Here's how the part is built. I have some questions about the finished solid (model axes, mm). Face numbers are marked on the shaded views. A direction names the side the tool comes from. Round coordinates to 2 decimals unless told otherwise and drop trailing zeros. Loops run counter-clockwise (first coordinate to the right, second up) from the corner with the lowest first, then second, coordinate; pieces in that order, holes last. Notation, with made-up numbers: M -16.75,5.5 L 11.25,5.5 A6 cw 11.25,13.5 Z; hole C 62.25,4 d10. An arc over 180 degrees is marked long. Answer as CSV lines item,"result".
```python
from build123d import *

# Parameters (mm, degrees)
F2_DEPTH = 12.7
F1_R     = 4.7625
F1_R_2   = 1.5875
F3_DEPTH = 9.525
F4_R     = 1.5875
F5_DEPTH = 15.859309


with BuildPart() as f2:
    # F0 (on Top) → F2 (new body)
    with BuildSketch(Plane.XY):
        with BuildLine():
            Line((-5.552635, 5.67205), (-5.552635, 8.681886))
            ThreePointArc((-5.552635, 8.681886), (0, -10.305673), (5.552635, 8.681886))
            Line((5.552635, 8.681886), (5.552635, 5.67205))
            ThreePointArc((5.552635, 5.67205), (7.317033, 3.076513), (7.9375, 0))
            ThreePointArc((7.9375, 0), (-3.076513, -7.317033), (-5.552635, 5.67205))
        make_face()
        with BuildLine():
            Line((-5.552635, 23.249359), (-5.552635, 8.681886))
            Line((-5.552635, 8.681886), (-5.552635, 5.67205))
            ThreePointArc((-5.552635, 5.67205), (-4.520661, 6.52438), (-3.360147, 7.191197))
            Line((-3.360147, 7.191197), (-3.360147, 23.249359))
            Line((-3.360147, 23.249359), (-5.552635, 23.249359))
        make_face()
        with BuildLine():
            Line((5.552635, 5.67205), (5.552635, 8.681886))
            Line((5.552635, 8.681886), (5.552635, 23.249359))
            Line((5.552635, 23.249359), (3.360147, 23.249359))
            Line((3.360147, 23.249359), (3.360147, 7.191197))
            ThreePointArc((3.360147, 7.191197), (4.520661, 6.52438), (5.552635, 5.67205))
        make_face()
    extrude(amount=F2_DEPTH)

    # F1 (on Right) → F3 (join, symmetric)
    with BuildSketch(Plane.YZ):
        with Locations((-12.700004, 4.7625)):
            Circle(F1_R)
        with Locations((-12.700004, 4.7625)):
            Circle(F1_R_2, mode=Mode.SUBTRACT)
    extrude(amount=F3_DEPTH, both=True)

    # F4 (on face) → F5 (cut, through all)
    with BuildSketch(Plane.YZ.offset(5.552635)):
        with Locations((15.965623, 6.35)):
            Circle(F4_R)
    extrude(amount=-F5_DEPTH, mode=Mode.SUBTRACT)


with BuildPart() as f6_1:
    # F6: copy of F2
    add(f2.part)


solid = f2.part
```
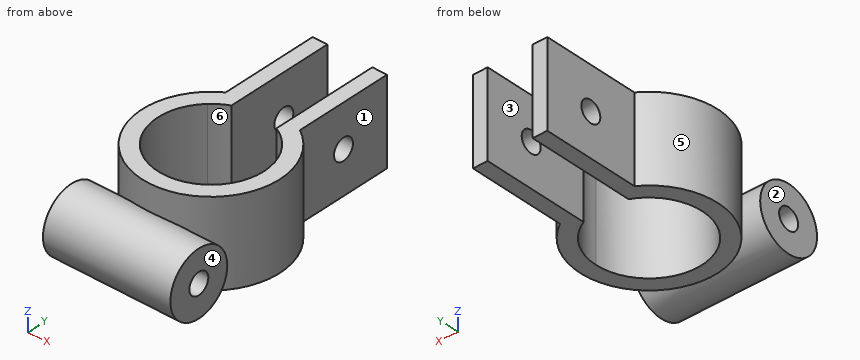
1. I want a section at B-B, the plane z = 11. Please give me the cut outline in (x, y) (1 decimal).
Evaluation:
outline,"M -5.6,5.7 A7.9 cw -3.4,7.2 L -3.4,23.2 L -5.6,23.2 L -5.6,8.7 A10.3 ccw long 5.6,8.7 L 5.6,23.2 L 3.4,23.2 L 3.4,7.2 A7.9 cw 5.6,5.7 A7.9 cw 7.9,0 A7.9 cw long Z"
2. I want a section at A-A, the plane x = -5. Count the separate pieces of the cut face and the enclosed holes in it, and give its area (3 significant figures).
Evaluation:
separate pieces,"2"
enclosed holes,"2"
area,"304 mm²"
3. We'd pull the mould along Y, two halves only. Please class the marked faces 4, 5 and 6: pulls with the +Y half, pulls with the -Y half, needs draft (parallel to the pull), parting line crosses it, or undercut.
Evaluation:
face 4,"needs draft"
face 5,"undercut"
face 6,"undercut"
4. Which directions (+Z, -Z, +X, -X, +Y, -Y) give clear straight access to the entire face, cutting with the end or side of a thin tool? Please do the marked faces 1, 2 and 3.
Evaluation:
face 1,"+Z, -Z, +X, +Y"
face 2,"+Z, -Z, -X, -Y"
face 3,"+Z, -Z, +Y"
5. If I drill on line 1 (X direction, y = 10, z = 10.5); line 2 (Y direction, x = -7, z = 6); line 3 (Y direction, x = 4, z = 5.75), over which ranges is the centre line in solid material (lowest first)? Write a range as [from, to].
Evaluation:
line 1,"x = [-5.55, -3.36], [3.36, 5.55]"
line 2,"y = [-17.3, -13.69], [-11.71, -8.1], [-7.56, -3.74], [3.74, 7.56]"
line 3,"y = [-17.36, -13.94], [-11.46, -6.86], [6.86, 14.5], [17.44, 23.25]"
6. I want a section at D-D, the plane z = 7.5. Please give me the cut outline in (x, y) (1 decimal).
Evaluation:
outline,"M -9.5,-16.6 L 9.5,-16.6 L 9.5,-8.8 L 5.4,-8.8 A10.3 ccw 5.6,8.7 L 5.6,14.9 L 3.4,14.9 L 3.4,7.2 A7.9 cw 5.6,5.7 A7.9 cw 7.9,0 A7.9 cw long -5.6,5.7 A7.9 cw -3.4,7.2 L -3.4,14.9 L -5.6,14.9 L -5.6,8.7 A10.3 ccw -5.4,-8.8 L -9.5,-8.8 Z; M -5.6,17.1 L -3.4,17.1 L -3.4,23.2 L -5.6,23.2 Z; M 3.4,17.1 L 5.6,17.1 L 5.6,23.2 L 3.4,23.2 Z"
7. For P1, Ø4, axis at y = 16.5, z = 4, coming from the -X side; P2, Ø5, axis at y = -6.5, z = 8, coming from the +X side (3 decimals); P3, Ø1, axis at y = -5, z = 7, coming from the +X side; P4, Ø1, axis at y = -11.5, z = 11, coming from the +X side, each with a flat end and sliding along its axis, tell me the tip position at first contact or that it passes through.
Evaluation:
P1,"stops at x = -5.55"
P2,"stops at x = 9.525"
P3,"stops at x = 9.27"
P4,"passes through"
8. I want a section at C-C, the plane x = -2. Please give me the cut outline in (y, z) (1 decimal).
Evaluation:
outline,"M -10.1,0 L -7.7,0 L -7.7,12.7 L -10.1,12.7 L -10.1,8.8 A4.8 ccw long -10.1,0.8 Z; hole C -12.7,4.8 d3.2"
